```python
from build123d import *

# Parameters (mm, degrees)
SKETCH1_R           = 12.5
BOSS_EXTRUDE1_DEPTH = 5
SKETCH2_R           = 4
BOSS_EXTRUDE2_DEPTH = 8
SKETCH3_W           = 5.51003513
SKETCH3_H           = 4.526021733
BOSS_EXTRUDE3_DEPTH = 6.5


with BuildPart() as part:
    # Sketch1 → Boss-Extrude1 (new body)
    with BuildSketch(Plane.XY):
        Circle(SKETCH1_R)
    extrude(amount=BOSS_EXTRUDE1_DEPTH)

    # Sketch2 → Boss-Extrude2 (add)
    with BuildSketch(Plane.XY.offset(5)):
        Circle(SKETCH2_R)
    extrude(amount=BOSS_EXTRUDE2_DEPTH)

    # Sketch3 → Boss-Extrude3 (add)
    with BuildSketch(Plane.XY.offset(13)):
        with Locations((0.009307382, -0.024270034)):
            Rectangle(SKETCH3_W, SKETCH3_H)
    extrude(amount=BOSS_EXTRUDE3_DEPTH)


solid = part.part
```
Here's how the part is built. I have some questions about the finished solid (model axes, mm). A direction names the side the tool comes from. Give positions to 0.01 mm unless a question says otherwise; leave off trailing zeros. Write each loop counter-clockwise with the first axis right and the second up, starting at its lowest first coordinate (ties: lowest second). Pieces come first, ordered by that corner, then holes.
(1) Imagine slicing it at C-C, the plane z = 6.75. Write out the boundary of the cut face in (x, y).
Output values:
outline: circle Ø8 at (0, 0)
(2) Imagine slicing it at D-D, the plane y = -3. Write out the boundary of the cut face in (x, z), and give its area (3 significant figures).
Output values:
outline: (-12.13, 0) - (12.13, 0) - (12.13, 5) - (2.65, 5) - (2.65, 13) - (-2.65, 13) - (-2.65, 5) - (-12.13, 5) - close
area: 164 mm2
(3) Imagine slicing it at B-B, the plane x = 0. Write out the boundary of the cut face in (y, z).
Output values:
outline: (-12.5, 0) - (12.5, 0) - (12.5, 5) - (4, 5) - (4, 13) - (2.24, 13) - (2.24, 19.5) - (-2.29, 19.5) - (-2.29, 13) - (-4, 13) - (-4, 5) - (-12.5, 5) - close
(4) If I drill on L1, parallel to Z at x = 5.5, y = 8.25; L2, parallel to Z at x = 0.5, y = -3.5; L3, parallel to X at y = -10.75, z = 3.75, over which ranges is the centre line in solid material (lowest first)?
Output values:
L1: z = 0 to 5
L2: z = 0 to 13
L3: x = -6.38 to 6.38
(5) Imagine slicing it at A-A, the plane y = 0. Write out the boundary of the cut face in (x, z), and give its area (3 significant figures).
Output values:
outline: (-12.5, 0) - (12.5, 0) - (12.5, 5) - (4, 5) - (4, 13) - (2.76, 13) - (2.76, 19.5) - (-2.75, 19.5) - (-2.75, 13) - (-4, 13) - (-4, 5) - (-12.5, 5) - close
area: 225 mm2
(6) On a 3-axis mill with a long thin cutter (end or side, diameter ignored), from which of +Z, -Z, +X, -X, +Y, -Y can I reach the whole of each face in a straight line? I mean faces 1 (the face through (0, -2.287, 16)), 2 (the face through (0, 2.239, 16)), 3 (the face through (2.764, 0, 16)), 4 (the face through (-3, 3, 5)). Say none if no direction works.
Output values:
face 1: +Z, +X, -X, -Y
face 2: +Z, +X, -X, +Y
face 3: +Z, +X, +Y, -Y
face 4: +Z
(7) Will these pins go through, and if not, where does the flat tip stop? pin 1 (4 mm diameter, centred on x = 9.5, y = -1.5, fed in from +Z); pin 2 (5 mm diameter, centred on y = -0.5, z = 16.5, fed in from -X); pin 3 (10 mm diameter, centred on x = -2, z = 8.5, fed in from +Y); pin 4 (4 mm diameter, centred on y = -7, z = 9, fed in from -X).
Output values:
pin 1: stops at z = 5
pin 2: stops at x = -2.75
pin 3: stops at y = 12.5
pin 4: passes through
